```python
from build123d import *

# Parameters (mm, degrees)
SKETCH096_W            = 300
SKETCH096_H            = 95
PAD053_DEPTH           = 5
SKETCH113_W            = 10
SKETCH113_H            = 5
PAD069_DEPTH           = 5
LINEARPATTERN065_COUNT = 5
LINEARPATTERN065_PITCH = 20
SKETCH114_W            = 10
SKETCH114_H            = 5
PAD070_DEPTH           = 5
LINEARPATTERN066_COUNT = 15
LINEARPATTERN066_PITCH = 20
SKETCH129_W            = 10
SKETCH129_H            = 5
PAD073_DEPTH           = 5
LINEARPATTERN081_COUNT = 15
LINEARPATTERN081_PITCH = 20


with BuildPart() as part:
    # Sketch096 → Pad053 (new body)
    with BuildSketch(Plane.XY):
        Rectangle(SKETCH096_W, SKETCH096_H)
    extrude(amount=PAD053_DEPTH)

    # Sketch113 (on DatumPlane) → Pad069 (join)
    with BuildSketch(Plane.YZ.offset(150)):
        with Locations((-37.5, 2.5)):
            Rectangle(SKETCH113_W, SKETCH113_H)
    pad069 = extrude(amount=PAD069_DEPTH)

    # LinearPattern065: Pad069 ×5
    with Locations(*[(0, i * LINEARPATTERN065_PITCH, 0) for i in range(1, LINEARPATTERN065_COUNT)]):
        add(pad069)

    # Sketch114 (on DatumPlane) → Pad070 (join)
    with BuildSketch(Plane.XZ.offset(47.5)):
        with Locations((-140, 2.5)):
            Rectangle(SKETCH114_W, SKETCH114_H)
    pad070 = extrude(amount=PAD070_DEPTH)

    # LinearPattern066: Pad070 ×15
    with Locations(*[(i * LINEARPATTERN066_PITCH, 0, 0) for i in range(1, LINEARPATTERN066_COUNT)]):
        add(pad070)

    # Sketch129 (on DatumPlane) → Pad073 (join)
    with BuildSketch(Plane(origin=(0, 47.5, 0), x_dir=(-1, 0, 0), z_dir=(0, 1, 0))):
        with Locations((-140, 2.5)):
            Rectangle(SKETCH129_W, SKETCH129_H)
    pad073 = extrude(amount=PAD073_DEPTH)

    # LinearPattern081: Pad073 ×15
    with Locations(*[(-i * LINEARPATTERN081_PITCH, 0, 0) for i in range(1, LINEARPATTERN081_COUNT)]):
        add(pad073)


with BuildPart() as part_1:
    # Body037 placement: moved
    add(part.part.moved(Location((-100, -97.5, 100))))


solid = part_1.part
```
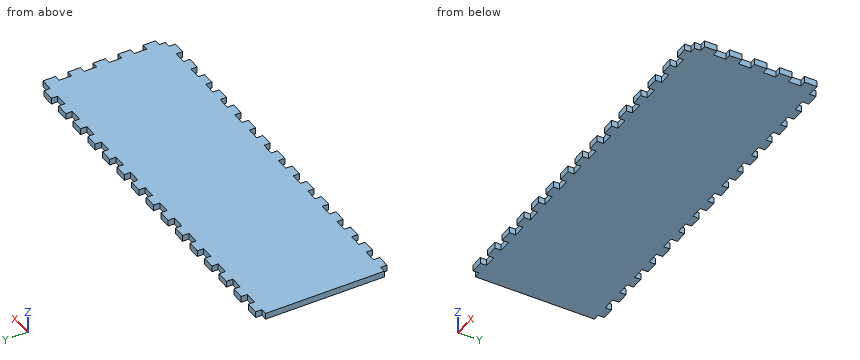
CAD build for the part. Positions are in the model's coordinates, mm. Give positions to 0.01 mm unless a question says otherwise; leave off trailing zeros. Order: outer loops, then holes, each group sorted by start corner. A loop starts at its lowest first (then second) coordinate and runs counter-clockwise, first axis right, second up.
(1) Drill centre lines: L1, parallel to X at y = -124, z = 102.1; L2, parallel to Y at x = -226.5, z = 104.45. Where is each one in solid material? Low to high.
(2) Flat gauge pins, fed straight in: pin 1 (2.5 mm diameter, centred on y = -147.5, z = 102.5, fed in from +X); pin 2 (2.5 mm diameter, centred on y = -147.5, z = 102, fed in from -X); pin 3 (1.5 mm diameter, centred on x = -29, z = 103.5, fed in from -Y). Where does each tip first touch, or does it go through?
(3) Saw through at A-A, the plane y = -85. Give the cut face in (x, z).
(4) Saw through at B-B, the plane x = -10.5. Give the cut face in (y, z).
Results found:
1. L1: x = -250 to 50
1. L2: y = -145 to -50
2. pin 1: stops at x = 45
2. pin 2: stops at x = -245
2. pin 3: stops at y = -145
3. outline: (-250, 100) - (50, 100) - (50, 105) - (-250, 105) - close
4. outline: (-145, 100) - (-50, 100) - (-50, 105) - (-145, 105) - close
